Verification items for the finished model (mm, model axes). A direction names the side the tool comes from. Coordinates: 2 decimals unless noted, no trailing zeros. Write each loop counter-clockwise with the first axis right and the second up, starting at its lowest first coordinate (ties: lowest second). Pieces come first, ordered by that corner, then holes. Notation, with made-up numbers: (72.5, 67.5) -> (125.5, 67.5) arc R21 cw to (125.5, 92.5) -> close; hole circle Ø9 at (-10.75, 88). An arc over 180 degrees is marked (long way). Use a Markdown table: item, result. Add a question column.
Autodesk Inventor part; units mm, degrees
ref_plane "YZ Plane" through (0, 0, 0) normal (1, 0, 0) x (0, 1, 0)
ref_plane "XZ Plane" through (0, 0, 0) normal (0, 1, 0) x (-1, 0, 0)
ref_plane "XY Plane" through (0, 0, 0) normal (0, 0, 1) x (1, 0, 0)
sketch "Sketch1" plane through (0, 0, 0) normal (0, 0, 1) x (1, 0, 0)
  line L0 (-22.6, -22.6) -> (22.6, -22.6)
  line L1 (22.6, -22.6) -> (22.6, 22.6)
  line L2 (22.6, 22.6) -> (-22.6, 22.6)
  line L3 (-22.6, 22.6) -> (-22.6, -22.6)
  line L4 (-22.6, -22.6) -> (22.6, 22.6) construction
  line L5 (22.6, -22.6) -> (20.5, -22.6) construction
  line L6 (20.5, -22.6) -> (20.4022, -20.4022) construction
  line L7 (20.4022, -20.4022) -> (-20.3978, -20.4022)
  line L8 (-20.3978, -20.4022) -> (-20.3978, -18.6022)
  line L9 (-20.3978, -18.6022) -> (20.4022, -18.6022)
  line L10 (20.4022, -18.6022) -> (20.4022, -20.4022)
  line L11 (-20.3978, -18.6022) -> (-18.5978, -18.6022)
  line L12 (-18.5978, -18.6022) -> (-18.5978, 20.3978)
  line L13 (-18.5978, 20.3978) -> (-20.3978, 20.3978)
  line L14 (-20.3978, 20.3978) -> (-20.3978, -18.6022)
  line L15 (-18.5978, 20.3978) -> (-17.3978, 20.3978)
  line L16 (-17.3978, 20.3978) -> (-17.3978, 14.5978)
  line L17 (-17.3978, 14.5978) -> (-18.5978, 14.5978)
  line L18 (-18.5978, 14.5978) -> (-18.5978, 20.3978)
  line L19 (20.4022, -18.6022) -> (14.6022, -18.6022)
  line L20 (14.6022, -18.6022) -> (14.6022, -17.4022)
  line L21 (14.6022, -17.4022) -> (20.4022, -17.4022)
  line L22 (20.4022, -17.4022) -> (20.4022, -18.6022)
  line L23 (22.6, 22.6) -> (-17.4, 22.6) construction
  line L24 (-17.4, 22.6) -> (-17.4, 14.6) construction
  line L25 (-17.4, 14.6) -> (22.6, 14.6) construction
  line L26 (22.6, 14.6) -> (22.6, 22.6) construction
  line L27 (22.6, 22.6) -> (14.6, 22.6) construction
  line L28 (14.6, 22.6) -> (14.6, -17.4) construction
  line L29 (14.6, -17.4) -> (22.6, -17.4) construction
  line L30 (22.6, -17.4) -> (22.6, 22.6) construction
  line L31 (14.6, 14.6) -> (-18.6, 14.6)
  line L32 (-18.6, 14.6) -> (-18.6, 12.6)
  line L33 (-18.6, 12.6) -> (14.6, 12.6)
  line L34 (14.6, 12.6) -> (14.6, 14.6)
  line L35 (14.6, 12.6) -> (12.6, 12.6)
  line L36 (12.6, 12.6) -> (12.6, -18.6)
  line L37 (12.6, -18.6) -> (14.6, -18.6)
  line L38 (14.6, -18.6) -> (14.6, 12.6)
  point P0 (0, 0)
  point P1 (-19.4978, 20.3978)
  point P2 (-17.3978, 14.6)
  point P3 (-18.5978, 12.6)
  dimension "d0" = 45.2
  dimension "d1" = 45.2
  dimension "d2" = 2.1
  dimension "d3" = 2.2
  dimension "d5" = 1.8
  dimension "d6" = 1.8
  dimension "d7" = 39
  dimension "d10" = 2.2022
  dimension "d11" = 4.0022
  dimension "d12" = 2.2022
  dimension "d15" = 1.2
  dimension "d16" = 5.8
  dimension "d21" = 5.8
  dimension "d22" = 1.2
  dimension "d25" = 40
  dimension "d26" = 8
  dimension "d27" = 8
  dimension "d28" = 40
  dimension "d29" = 33.2
  dimension "d30" = 2
  dimension "d31" = 2
  dimension "d32" = 31.2
extrude "Extrusion1" add sketch "Sketch1" along normal blind 3 contours L7 L8 L9 L10 | L14 L13 L12 L31 L32 L33 L9 | L33 L32 L31 L12
extrude "Extrusion2" add sketch "Sketch1" against normal blind 2 contours L3 L2 L1 L0 | L7 L8 L9 L10 | L9 L20 L21 L22 | L14 L13 L12 L31 L32 L33 L9 | L33 L32 L31 L12 | L12 L17 L16 L31 L34 L33 | L15 L16 L31 L12 | L12 L31 L16 L17 | L33 L38 L37 L36
extrude "Extrusion4" add sketch "Sketch1" along normal blind 3 contours L9 L20 L21 L22 | L15 L16 L31 L12 | L12 L31 L16 L17
extrude "Extrusion5" add sketch "Sketch1" along normal blind 3 contours L12 L17 L16 L31 L34 L33 | L33 L38 L37 L36
fillet "Fillet1" radius 1 1 edges at (-22.6, -22.6, -1)
properties part number "DownCover" material "ABS Plastic"
1) Release check for a two-part mould opening along X. For faces 1 (the face through (-17.398, 18, 1)), 2 (the face through (-18.598, -3, 1)), 3 (the face through (-22.6, 1, -1)), 4 (the face through (-2, -18.602, 1)) record: released by +X, released by -X, zero draft, split by the parting line, or undercut.
2) Cross-section at C-C on z = 1.5. Record the boundary of the cut face in (x, y), then the cut area to 3 significant figures.
3) Cross-section at B-B on x = 6.5. Record the boundary of the cut face in (y, z).
4) Gauge pin test, flat ends, axial feed: pin 1 (1.5 mm diameter, centred on y = -9, z = 1, fed in from -X); pin 2 (1.5 mm diameter, centred on y = -9.5, z = 1.5, fed in from +X); pin 3 (1 mm diameter, centred on x = -13.5, z = 2.5, fed in from -Y). Record the tip position at first contact, or that the pin passes through.
5) Thickness scan on L1, parallel to Y at x = -4, z = 0.35; L2, parallel to Z at x = -2, y = -9. Record the ranges inside material, lowest first.
6) Cross-section at A-A on y = 14. Record the boundary of the cut face in (x, z).
7) Set-up check for faces 5 (the face through (17, -17.402, 1)), 6 (the face through (0, -20.402, 1)), 7 (the face through (20.402, -19, 1)): record each of +Z, -Z, +X, -X, +Y, -Y from which the full face is reachable in a straight line by a thin tool's end or side.
Returned:
| question | item | result |
|---|---|---|
| 1 | face 1 | released by +X |
| 1 | face 2 | undercut |
| 1 | face 3 | released by -X |
| 1 | face 4 | undercut |
| 2 | outline | (-20.4, -20.4) -> (20.4, -20.4) -> (20.4, -17.4) -> (14.6, -17.4) -> (14.6, -18.6) -> (-18.6, -18.6) -> (-18.6, 12.6) -> (12.6, 12.6) -> (12.6, -18.6) -> (14.6, -18.6) -> (14.6, 14.6) -> (-17.4, 14.6) -> (-17.4, 20.4) -> (-20.4, 20.4) -> close |
| 2 | area | 286 mm² |
| 3 | outline | (-22.6, -2) -> (22.6, -2) -> (22.6, 0) -> (14.6, 0) -> (14.6, 3) -> (12.6, 3) -> (12.6, 0) -> (-18.6, 0) -> (-18.6, 3) -> (-20.4, 3) -> (-20.4, 0) -> (-22.6, 0) -> close |
| 4 | pin 1 | stops at x = -20.4 |
| 4 | pin 2 | stops at x = 14.6 |
| 4 | pin 3 | stops at y = -20.4 |
| 5 | L1 | y = -20.4 to -18.6, 12.6 to 14.6 |
| 5 | L2 | z = -2 to 0 |
| 6 | outline | (-22.6, -2) -> (22.6, -2) -> (22.6, 0) -> (14.6, 0) -> (14.6, 3) -> (-20.4, 3) -> (-20.4, 0) -> (-22.6, 0) -> close |
| 7 | face 5 | +Z, +X, +Y |
| 7 | face 6 | +Z, +X, -X, -Y |
| 7 | face 7 | +Z, +X, +Y, -Y |
